For this review, use the dimensioned drawing (mm, ordinates from the lowest corner) and the shaded views. A direction names the side the tool comes from. Give positions to 0.01 mm unless a question says otherwise; leave off trailing zeros. Order: outer loops, then holes, each group sorted by start corner. A loop starts at its lowest first (then second) coordinate and runs counter-clockwise, first axis right, second up. Notation, with made-up numbers: M -22,22.25 L 4,22.25 A20 cw 4,47.25 Z; hole C 39.5,61 d3. An arc over 180 degrees is marked long. One line per question, with ' | ' between items. Start each with the question number.
1. Insertion check: P1, Ø3, axis at x = 5, y = 14.5, coming from the +Z side; P2, Ø2.5, axis at y = 9.5, z = 3.5, coming from the +X side; P3, Ø12, axis at y = 17.5, z = 12, coming from the -X side; P4, Ø1.5, axis at x = 21.5, y = 17, coming from the +Z side. Each pin has a flat end and moves straight along its axis. Give the tip position at first contact, or say it passes through.
2. The part is to be moulded in two halves that separate along Z. For the marked faces 1, 2 and 3, say which applies: +Z half, -Z half, draft (parallel to the pull), parting line (faces both ways), or undercut.
3. We need section A-A on z = 1.5. Write out the cut boundary in (x, y).
4. We need section B-B on y = 1.5. Write out the cut boundary in (x, z).
5. For the marked faces 4 and 5, list the 3-axis set-ups (+Z, -Z, +X, -X, +Y, -Y) from which the entire face can be reached by the end or side of a thin tool; tool diameter is ignored.
6. We need section D-D on x = 18.5. Write out the cut boundary in (y, z) (1 decimal).
7. Wall thickness on L1, parallel to X at y = 14.5, z = 2.5; L2, parallel to Y at x = 10.5, z = 14.5; L3, parallel to Z at x = 20, y = 11.75: over which ranges is each line inside the solid? List them lowest first.
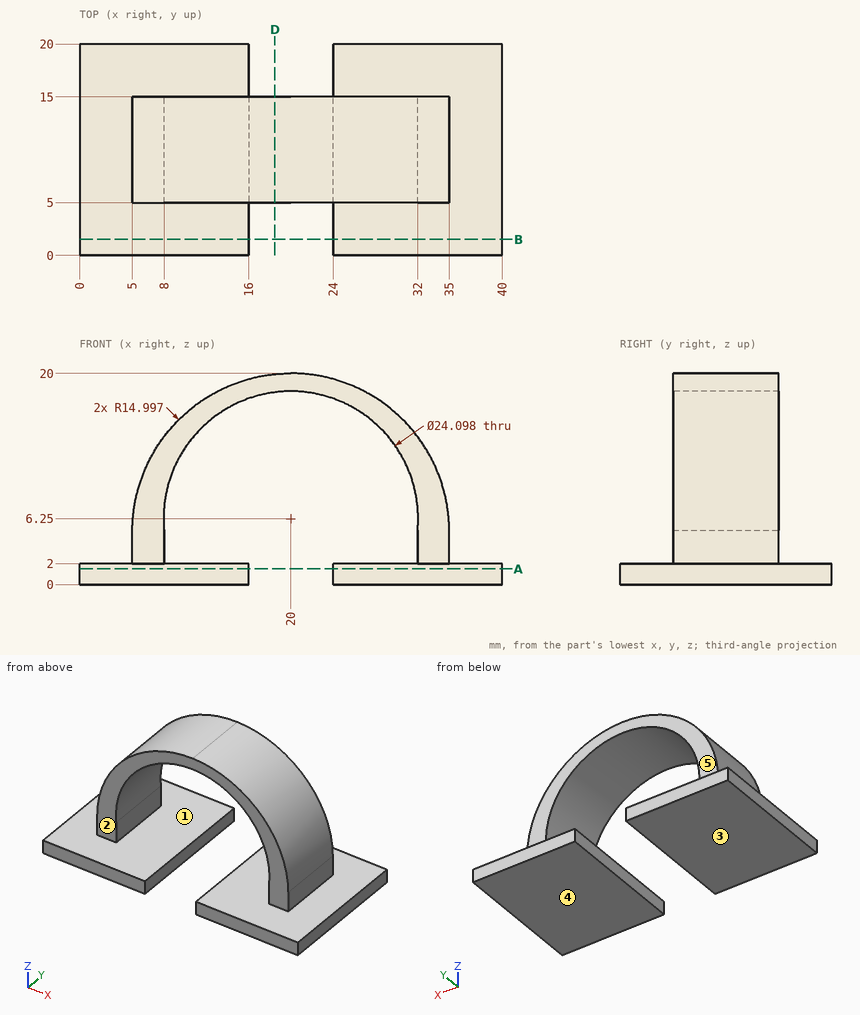
Entries:
1) P1: stops at z = 11.54 | P2: stops at x = 35 | P3: stops at x = 5.08 | P4: passes through
2) face 1: undercut | face 2: draft | face 3: -Z half
3) outline: M 0,0 L 16,0 L 16,20 L 0,20 Z; M 24,0 L 40,0 L 40,20 L 24,20 Z
4) outline: M 0,0 L 16,0 L 16,2 L 0,2 Z; M 24,0 L 40,0 L 40,2 L 24,2 Z
5) face 4: -Z, +X, -X, +Y, -Y | face 5: +Z, +X, -X, +Y
6) outline: M 5,18.2 L 15,18.2 L 15,19.9 L 5,19.9 Z
7) L1: x = 5 to 8, 32 to 35 | L2: y = 5 to 15 | L3: z = 18.3 to 20
